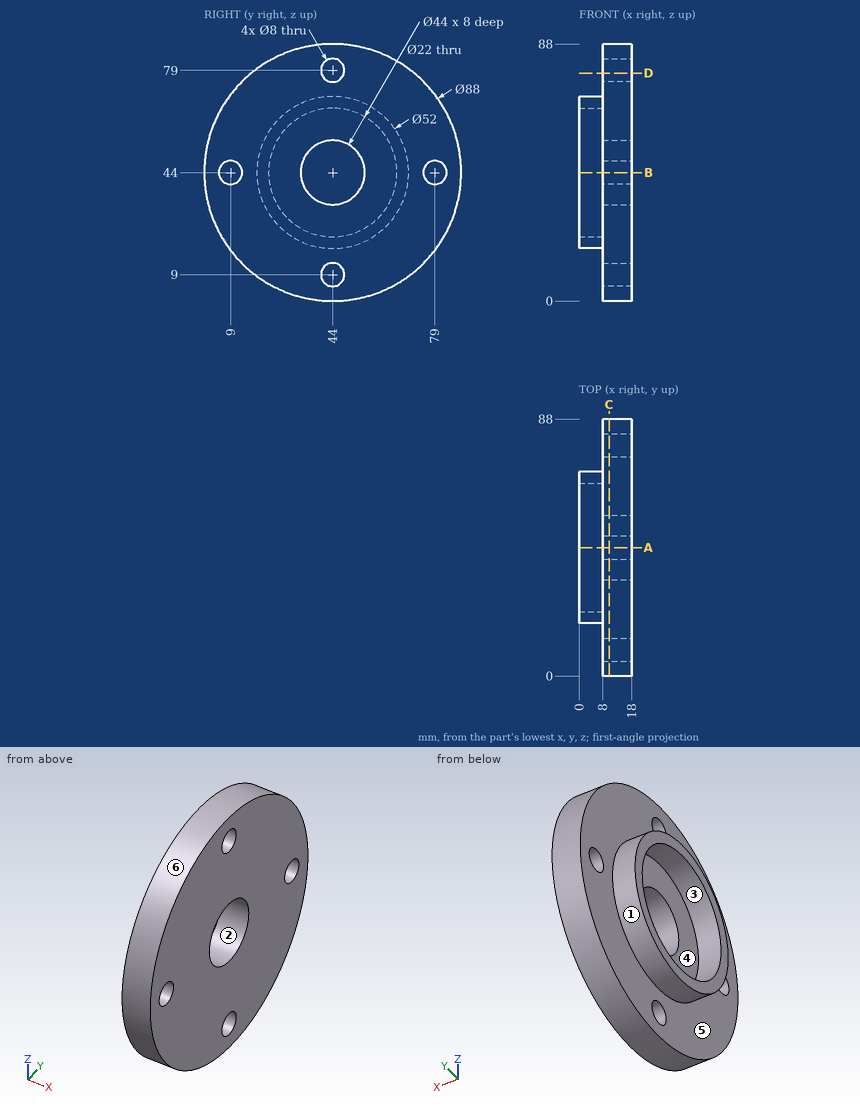
Here's the drawing with two shaded views (mm, measured from the low corner). I have some questions. A direction names the side the tool comes from. Round coordinates to 2 decimals unless told otherwise and drop trailing zeros. Order: outer loops, then holes, each group sorted by start corner. A loop starts at its lowest first (then second) coordinate and runs counter-clockwise, first axis right, second up. Notation, with made-up numbers: M -9,11.25 L 2,11.25 A26 ccw 2,46.25 Z; hole C 20,80 d5. An arc over 180 degrees is marked long. Answer in a Markdown table with one row per item.
Item 1: Imagine slicing it at A-A, the plane y = 44. Write out the boundary of the cut face in (x, z), and give its area (3 significant figures).
A:
| item | result |
|---|---|
| outline | M 0,18 L 8,18 L 8,13 L 18,13 L 18,33 L 8,33 L 8,22 L 0,22 Z; M 0,66 L 8,66 L 8,55 L 18,55 L 18,75 L 8,75 L 8,70 L 0,70 Z; M 8,0 L 18,0 L 18,5 L 8,5 Z; M 8,83 L 18,83 L 18,88 L 8,88 Z |
| area | 564 mm2 |
Item 2: Imagine slicing it at D-D, the plane z = 78. Write out the boundary of the cut face in (x, y), and give its area (3 significant figures).
A:
| item | result |
|---|---|
| outline | M 8,16.07 L 18,16.07 L 18,40.13 L 8,40.13 Z; M 8,47.87 L 18,47.87 L 18,71.93 L 8,71.93 Z |
| area | 481 mm2 |
Item 3: Imagine slicing it at C-C, the plane x = 10.25. Write out the boundary of the cut face in (y, z).
A:
| item | result |
|---|---|
| outline | C 44,44 d88; hole C 9,44 d8; hole C 44,44 d22; hole C 44,9 d8; hole C 44,79 d8; hole C 79,44 d8 |
Item 4: I'm going to push flat-ended pins straight in: pin 1 (6 mm diameter, centred on x = 7.5, z = 64.5, fed in from +Y); pin 2 (10 mm diameter, centred on x = 9, y = 74, fed in from +Z); pin 3 (20 mm diameter, centred on y = 44, z = 44, fed in from -X); pin 4 (1 mm diameter, centred on y = 26, z = 37, fed in from -X). Where does each tip first touch, or does it pass through?
A:
| item | result |
|---|---|
| pin 1 | stops at y = 84.35 |
| pin 2 | stops at z = 80.21 |
| pin 3 | passes through |
| pin 4 | stops at x = 8 |
Item 5: Thinking about a two-plate mould opening in Z: for the marked faces 3, 4, 5 and 6, which applies, +Z half, -Z half, draft (parallel to the pull), parting line (faces both ways), or undercut?
A:
| item | result |
|---|---|
| face 3 | undercut |
| face 4 | undercut |
| face 5 | draft |
| face 6 | parting line |
Item 6: For the marked faces 1 and 2, which set-ups out of +Z, -Z, +X, -X, +Y, -Y let a thin tool reach every point of the face, with its end or its side?
A:
| item | result |
|---|---|
| face 1 | -X |
| face 2 | +X, -X |
Item 7: If I drill on L1, parallel to Y at x = 12, z = 44; L2, parallel to Y at x = 5, z = 44; L3, parallel to X at y = 81, z = 37, over which ranges is the centre line in solid material (lowest first)? Write a range as from..to.
A:
| item | result |
|---|---|
| L1 | y = 0..5, 13..33, 55..75, 83..88 |
| L2 | y = 18..22, 66..70 |
| L3 | x = 8..18 |
